Source: CAD feature listing. Evaluate the final solid. Frame: model axes, mm. Face numbers are marked on the shaded views. A direction names the side the tool comes from. Give positions to 0.01 mm unless a question says otherwise; leave off trailing zeros. Order: outer loops, then holes, each group sorted by start corner. A loop starts at its lowest first (then second) coordinate and runs counter-clockwise, first axis right, second up. Notation, with made-up numbers: (55.25, -37.5) -> (102.25, -37.5) arc R5 cw to (102.25, -29.5) -> close; hole circle Ø2 at (-1, 41). An arc over 180 degrees is marked (long way). Answer in a Markdown table with one row per item.
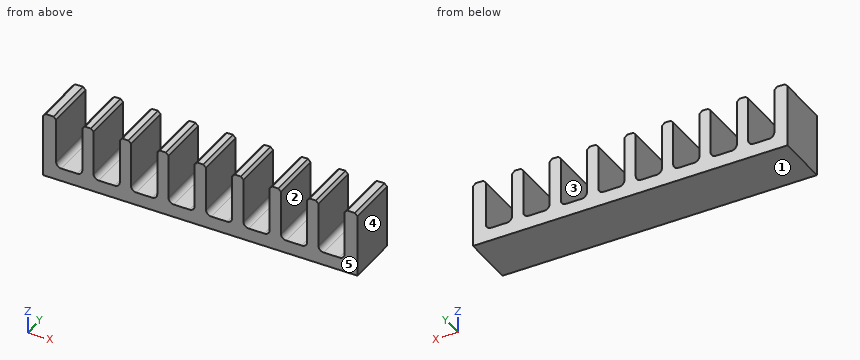
```python
from build123d import *

# Parameters (mm, degrees)
F0_W     = 152.4
F0_H     = 25.4
F1_DEPTH = 31.75
F2_W     = 12.7
F2_H     = 25.4
F3_DEPTH = 25.401
F4_R     = 2.54
F5_SIZE  = 1.27


with BuildPart() as f1:
    # F0 (on Top) → F1 (new body)
    with BuildSketch(Plane.XY):
        Rectangle(F0_W, F0_H)
    extrude(amount=F1_DEPTH)

    # F2 (on face) → F3 (cut, through all)
    with BuildSketch(Plane.XZ.offset(12.7)):
        with Locations((-63.5, 19.05)):
            Rectangle(F2_W, F2_H)
        with Locations((-45.339, 19.05)):
            Rectangle(F2_W, F2_H)
        with Locations((-27.178, 19.05)):
            Rectangle(F2_W, F2_H)
        with Locations((-9.017, 19.05)):
            Rectangle(F2_W, F2_H)
        with Locations((9.144, 19.05)):
            Rectangle(F2_W, F2_H)
        with Locations((27.305, 19.05)):
            Rectangle(F2_W, F2_H)
        with Locations((45.466, 19.05)):
            Rectangle(F2_W, F2_H)
        with Locations((63.627, 19.05)):
            Rectangle(F2_W, F2_H)
    extrude(amount=-F3_DEPTH, mode=Mode.SUBTRACT)

    # F4
    f4_edges = [f1.edges().sort_by_distance(p)[0] for p in [
        (-69.85, 0, 6.35),
        (-57.15, 0, 6.35),
        (-38.989, 0, 6.35),
        (-20.828, 0, 6.35),
        (-2.667, 0, 6.35),
        (15.494, 0, 6.35),
        (33.655, 0, 6.35),
        (51.816, 0, 6.35),
        (69.977, 0, 6.35),
        (57.277, 0, 6.35),
        (39.116, 0, 6.35),
        (20.955, 0, 6.35),
        (2.794, 0, 6.35),
        (-15.367, 0, 6.35),
        (-33.528, 0, 6.35),
        (-51.689, 0, 6.35),
    ]]
    fillet(f4_edges, radius=F4_R)

    # F5
    f5_edges = [f1.edges().sort_by_distance(p)[0] for p in [
        (-69.85, 0, 31.75),
        (-76.2, 0, 31.75),
        (-57.15, 0, 31.75),
        (-51.689, 0, 31.75),
        (-38.989, 0, 31.75),
        (-33.528, 0, 31.75),
        (-20.828, 0, 31.75),
        (-15.367, 0, 31.75),
        (-2.667, 0, 31.75),
        (2.794, 0, 31.75),
        (15.494, 0, 31.75),
        (20.955, 0, 31.75),
        (33.655, 0, 31.75),
        (39.116, 0, 31.75),
        (51.816, 0, 31.75),
        (57.277, 0, 31.75),
        (69.977, 0, 31.75),
        (76.2, 0, 31.75),
    ]]
    chamfer(f5_edges, length=F5_SIZE)


solid = f1.part
```
(1) Access query for the marked faces 1 and 2. Directions: +Z, -Z, +X, -X, +Y, -Y. A direction counts if a zero-diameter tool reaches every point of the face in a straight line with its end or side. Return the directions, or none.
A:
| item | result |
|---|---|
| face 1 | -Z, +X, -X, +Y, -Y |
| face 2 | +Z, +Y, -Y |
(2) Ray query, probe 1 along Z at (x, y) = (42, -7.25); probe 2 along Z at (x, y) = (21.5, 3). Return the intervals inside material, ascending.
A:
| item | result |
|---|---|
| probe 1 | z = 0 to 6.35 |
| probe 2 | z = 0 to 7.32 |
(3) Section query B-B (x = 44.5). Return the cut outline in (y, z), plus the area to 3 significant figures.
A:
| item | result |
|---|---|
| outline | (-12.7, 0) -> (12.7, 0) -> (12.7, 6.35) -> (-12.7, 6.35) -> close |
| area | 161 mm^2 |
(4) First-contact query: pin 1 Ø4 at (x, y) = (25.5, 2) entering from +Z; pin 2 Ø6 at (x, y) = (47, 4.5) entering from +Z; pin 3 Ø6 at (x, y) = (-36.5, -5.5) entering from -Z; pin 4 Ø6 at (x, z) = (-12, 21.5) entering from +Y. Flat tips, straight axial feed; report the tip coordinate or a pass-through.
A:
| item | result |
|---|---|
| pin 1 | stops at z = 6.35 |
| pin 2 | stops at z = 6.46 |
| pin 3 | stops at z = 0 |
| pin 4 | passes through |
(5) Pull-direction query (X, two-part tool) for the marked faces 3, 4 and 5; classes: +X half, -X half, draft (parallel to the pull), parting line (faces both ways), or undercut.
A:
| item | result |
|---|---|
| face 3 | undercut |
| face 4 | +X half |
| face 5 | draft |
(6) Section query A-A (z = 20). Give the number of separate pieces and of enclosed holes in the cut face, plus the area to 3 significant figures.
A:
| item | result |
|---|---|
| separate pieces | 9 |
| enclosed holes | 0 |
| area | 1,290 mm^2 |
